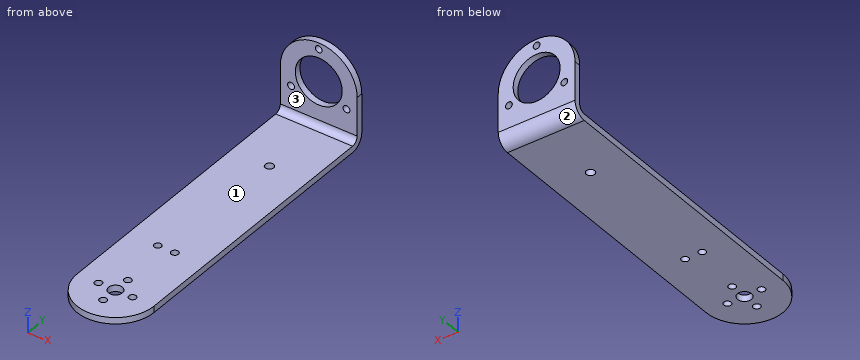
from build123d import *

# Parameters (mm, degrees)
SKETCH_1_R                                 = 3.25
SKETCH_1_R_2                               = 1.7
SKETCH_1_R_3                               = 2
F_01_MAIN_PLATE_135_W36_T3_EST_HOLES_DEPTH = 3
SKETCH_2_R                                 = 11
SKETCH_2_R_2                               = 1.6
F_02_FLANGE_H42_HOLE22_EST_DEPTH           = 3
F_03_BEND_INNER_R3_EST_R                   = 3
F_04_BEND_OUTER_R6_EST_R                   = 6


with BuildPart() as part:
    # 草图1 → 01_Main_plate_135_W36_T3_EST_holes (new body)
    with BuildSketch(Plane.XY):
        with BuildLine():
            Line((-18, 0), (-18, 135))
            Line((-18, 135), (18, 135))
            Line((18, 135), (18, 0))
            ThreePointArc((18, 0), (0, -18), (-18, 0))
        make_face()
        Circle(SKETCH_1_R, mode=Mode.SUBTRACT)
        with Locations((-8, 0)):
            Circle(SKETCH_1_R_2, mode=Mode.SUBTRACT)
        with Locations((8, 0)):
            Circle(SKETCH_1_R_2, mode=Mode.SUBTRACT)
        with Locations((0, -8)):
            Circle(SKETCH_1_R_2, mode=Mode.SUBTRACT)
        with Locations((0, 8)):
            Circle(SKETCH_1_R_2, mode=Mode.SUBTRACT)
        with Locations((-4, 33)):
            Circle(SKETCH_1_R_2, mode=Mode.SUBTRACT)
        with Locations((4, 33)):
            Circle(SKETCH_1_R_2, mode=Mode.SUBTRACT)
        with Locations((0, 100)):
            Circle(SKETCH_1_R_3, mode=Mode.SUBTRACT)
    extrude(amount=F_01_MAIN_PLATE_135_W36_T3_EST_HOLES_DEPTH)

    # 草图2 → 02_Flange_H42_hole22_EST (add)
    with BuildSketch(Plane(origin=(0, 135, 0), x_dir=(1, 0, 0), z_dir=(0, 1, 0))):
        with BuildLine():
            Line((-18, 0), (18, 0))
            Line((18, 0), (18, -24))
            ThreePointArc((18, -24), (0, -42), (-18, -24))
            Line((-18, -24), (-18, 0))
        make_face()
        with Locations(Location((0, -24, 0), (0, 0, 270))):
            Circle(SKETCH_2_R, mode=Mode.SUBTRACT)
        with Locations(Location((0, -39, 0), (0, 0, 270))):
            Circle(SKETCH_2_R_2, mode=Mode.SUBTRACT)
        with Locations(Location((-12.990381, -16.5, 0), (0, 0, 270))):
            Circle(SKETCH_2_R_2, mode=Mode.SUBTRACT)
        with Locations(Location((12.990381, -16.5, 0), (0, 0, 270))):
            Circle(SKETCH_2_R_2, mode=Mode.SUBTRACT)
    extrude(amount=-F_02_FLANGE_H42_HOLE22_EST_DEPTH)

    # 03_Bend_inner_R3_EST
    f_03_bend_inner_r3_est_edges = [part.edges().sort_by_distance(p)[0] for p in [
        (0, 132, 3),
    ]]
    fillet(f_03_bend_inner_r3_est_edges, radius=F_03_BEND_INNER_R3_EST_R)

    # 04_Bend_outer_R6_EST
    f_04_bend_outer_r6_est_edges = [part.edges().sort_by_distance(p)[0] for p in [
        (0, 135, 0),
    ]]
    fillet(f_04_bend_outer_r6_est_edges, radius=F_04_BEND_OUTER_R6_EST_R)


solid = part.part
Verification items for the finished model (mm, model axes). Face numbers are marked on the shaded views. Give positions to 0.01 mm unless a question says otherwise; leave off trailing zeros. Loops run counter-clockwise (first coordinate to the right, second up) from the corner with the lowest first, then second, coordinate; pieces in that order, holes last.
1. Cross-section at A-A on y = 8. Record the cut outline in (x, z).
Derived:
outline: (-18, 0) - (-1.7, 0) - (-1.7, 3) - (-18, 3) - close; (1.7, 0) - (18, 0) - (18, 3) - (1.7, 3) - close
2. Cross-section at D-D on x = -8. Record the cut outline in (y, z), and give its area (3 significant figures).
Derived:
outline: (-16.12, 0) - (-1.7, 0) - (-1.7, 3) - (-16.12, 3) - close; (1.7, 0) - (129, 0) arc R6 ccw to (135, 6) - (135, 16.45) - (132, 16.45) - (132, 6) arc R3 cw to (129, 3) - (1.7, 3) - close; (132, 31.55) - (135, 31.55) - (135, 40.12) - (132, 40.12) - close
area: 503 mm2
3. Release check for a two-part mould opening along Y. For the marked faces 1, 2 and 3 record: +Y half, -Y half, draft (parallel to the pull), parting line (faces both ways), or undercut.
Derived:
face 1: draft
face 2: +Y half
face 3: -Y half
4. Cross-section at C-C on z = 16.5. Record the cut outline in (x, y).
Derived:
outline: (-18, 132) - (-14.59, 132) - (-14.59, 135) - (-18, 135) - close; (-11.39, 132) - (-8.05, 132) - (-8.05, 135) - (-11.39, 135) - close; (8.05, 132) - (11.39, 132) - (11.39, 135) - (8.05, 135) - close; (14.59, 132) - (18, 132) - (18, 135) - (14.59, 135) - close
5. Material ranges on probe 1 along Y at (x, z) = (0, 0.85); probe 2 along Z at (x, y) = (1, -5); probe 3 along Y at (x, z) = (-3, 7), recorded low to high.
Derived:
probe 1: y = -18 to -9.7, -6.3 to -3.25, 3.25 to 6.3, 9.7 to 98, 102 to 132.08
probe 2: z = 0 to 3
probe 3: y = 132 to 135
6. Cross-section at B-B on x = 0. Count the separate pieces of the cut face and the enclosed holes in it, and give its area (3 significant figures).
Derived:
separate pieces: 7
enclosed holes: 0
area: 443 mm2
7. Go/stop test with flat-tipped pins: P1, Ø5.5, axis at x = 8, y = 0, coming from the +Z side; P2, Ø3, axis at x = 4, y = 33, coming from the +Z side (3 decimals); P3, Ø5, axis at x = 2.5, z = 37.5, coming from the -Y side. Record where each tip stops, or that it passes through.
Derived:
P1: stops at z = 3
P2: passes through
P3: stops at y = 132
